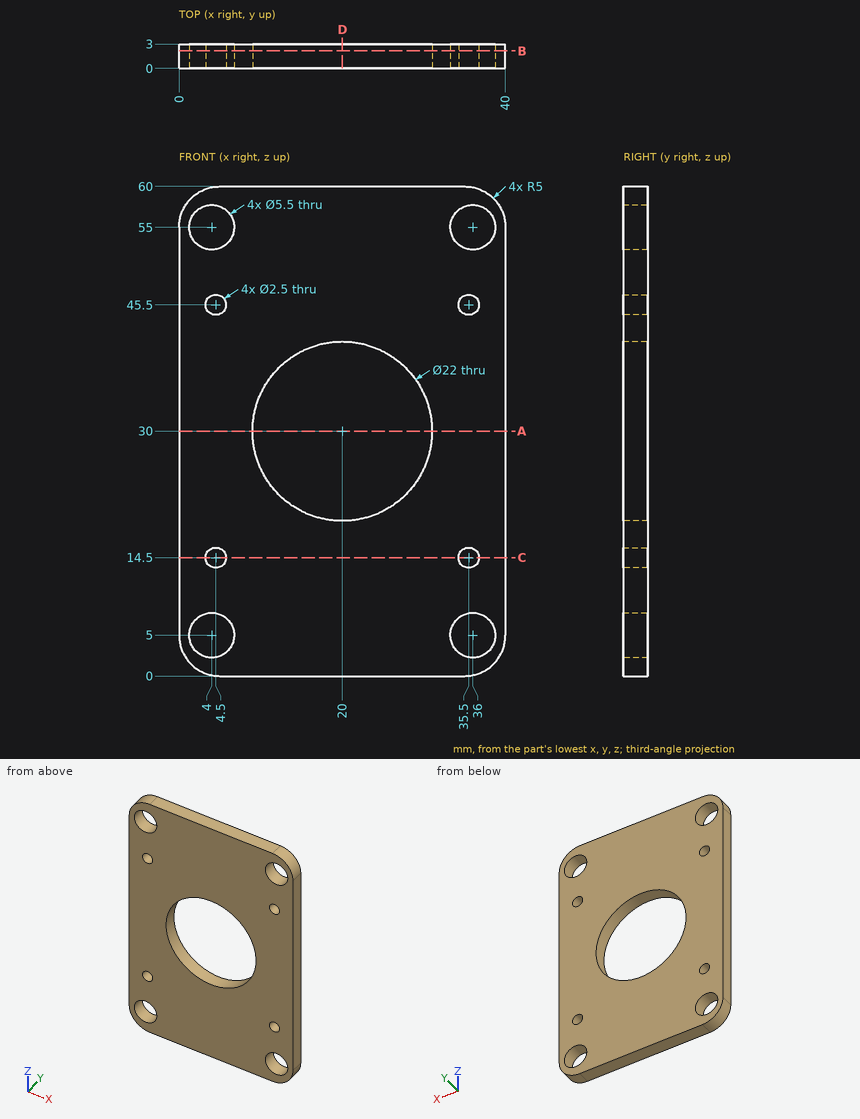
Here's the drawing with two shaded views (mm, measured from the low corner). I have some questions. Give positions to 0.01 mm unless a question says otherwise; leave off trailing zeros. Write each loop counter-clockwise with the first axis right and the second up, starting at its lowest first coordinate (ties: lowest second). Pieces come first, ordered by that corner, then holes. Notation, with made-up numbers: (47.5, 54) -> (84.5, 54) arc R15 cw to (84.5, 59) -> close; hole circle Ø10 at (67, 58). An arc over 180 degrees is marked (long way). Use one line per item in the form item = value.
1) Suppose I cut it at D-D (x = 20). Please give me the cut outline in (y, z), and give its area (3 significant figures).
Verdict:
outline = (0, 0) -> (3, 0) -> (3, 19) -> (0, 19) -> close; (0, 41) -> (3, 41) -> (3, 60) -> (0, 60) -> close
area = 114 mm2
2) Suppose I cut it at B-B (y = 2.15). Give the number of separate pieces and of enclosed holes in the cut face, and give its area (3 significant figures).
Verdict:
separate_pieces = 1
enclosed_holes = 9
area = 1,880 mm2
3) Suppose I cut it at A-A (z = 30). Please give me the cut outline in (x, y), and give its area (3 significant figures).
Verdict:
outline = (0, 0) -> (9, 0) -> (9, 3) -> (0, 3) -> close; (31, 0) -> (40, 0) -> (40, 3) -> (31, 3) -> close
area = 54.0 mm2
4) If I drill on L1, parallel to X at y = 0.75, z = 45.5; L2, parallel to X at y = 0.95, z = 55; L3, parallel to Z at x = 6.5, y = 2.45, over which ranges is the centre line in solid material (lowest first)? Write a range as [from, to].
Verdict:
L1 = [0, 3.25], [5.75, 34.25], [36.75, 40]
L2 = [0, 1.25], [6.75, 33.25], [38.75, 40]
L3 = [0, 3.85], [6.15, 53.85], [56.15, 60]
5) Suppose I cut it at C-C (z = 14.5). Please give me the cut outline in (x, y), and give its area (3 significant figures).
Verdict:
outline = (0, 0) -> (3.25, 0) -> (3.25, 3) -> (0, 3) -> close; (5.75, 0) -> (34.25, 0) -> (34.25, 3) -> (5.75, 3) -> close; (36.75, 0) -> (40, 0) -> (40, 3) -> (36.75, 3) -> close
area = 105 mm2
